Autodesk Inventor part; units mm, degrees
ref_plane "YZ Plane" through (0, 0, 0) normal (1, 0, 0) x (0, 1, 0)
ref_plane "XZ Plane" through (0, 0, 0) normal (0, 1, 0) x (-1, 0, 0)
ref_plane "XY Plane" through (0, 0, 0) normal (0, 0, 1) x (1, 0, 0)
sketch "Sketch1" plane through (0, 0, 0) normal (0, 0, 1) x (1, 0, 0)
  circle A0 centre (15, -15) radius 1.2295
  circle A1 centre (-15, 15) radius 1.2295
  circle A2 centre (15, 15) radius 1.2295
  circle A3 centre (-15, -15) radius 1.2295
  line L0 (-15.5, -17.5) -> (-17.5, -15.5)
  line L1 (-15.5, -17.5) -> (15.5, -17.5)
  line L2 (17.5, -15.5) -> (15.5, -17.5)
  line L3 (17.5, -15.5) -> (17.5, 15.5)
  line L4 (15.5, 17.5) -> (17.5, 15.5)
  line L5 (15.5, 17.5) -> (-15.5, 17.5)
  line L6 (-17.5, 15.5) -> (-15.5, 17.5)
  line L7 (-17.5, 15.5) -> (-17.5, -15.5)
  point P0 (0, 0)
  point P1 (0, 0)
  point P2 (0, 0)
extrude "Extrusion1" add sketch "Sketch1" along normal mid plane 7.5
sketch "Sketch4" plane through (0, 0, -3.75) normal (0, 0, -1) x (-1, 0, 0)
  line L0 (-13.25, 13.25) -> (13.25, 13.25)
  line L1 (13.25, 13.25) -> (13.25, -13.25)
  line L2 (13.25, -13.25) -> (-13.25, -13.25)
  line L3 (-13.25, -13.25) -> (-13.25, 13.25)
  line L4 (-17.5, 15.5) -> (-17.5, -15.5)
  line L5 (15.5, 17.5) -> (-15.5, 17.5)
  point P0 (0, 0)
  point P1 (-13.25, 0)
  point P2 (0, 13.25)
  dimension "d15" = 4.25
  dimension "d16" = 4.25
extrude "Extrusion4" add sketch "Sketch4" along normal blind 12.5
sketch "Sketch5" plane through (0, 0, 3.75) normal (0, 0, 1) x (1, 0, 0)
  line L0 (13.25, -13.25) -> (-13.25, -13.25)
  line L1 (-13.25, -13.25) -> (-13.25, 13.25)
  line L2 (-13.25, 13.25) -> (13.25, 13.25)
  line L3 (13.25, 13.25) -> (13.25, -13.25)
  line L4 (-11.25, -11.25) -> (11.25, -11.25)
  line L5 (11.25, -11.25) -> (11.25, 11.25)
  line L6 (11.25, 11.25) -> (-11.25, 11.25)
  line L7 (-11.25, 11.25) -> (-11.25, -11.25)
  point P0 (0, 0)
  dimension "d19" = 2
extrude "Extrusion5" cut sketch "Sketch5" against normal blind 12.5 contours L7 L6 L5 L4
fillet "Fillet2" radius 2 4 edges at (11.25, 0, 3.75) (-11.25, 0, 3.75) (0, 11.25, 3.75) (0, -11.25, 3.75)
chamfer "Chamfer2" distance 2 angle 45 8 edges at (13.25, -13.25, -10) (13.25, 13.25, -10) (-13.25, -13.25, -10) (-13.25, 13.25, -10) (0, -13.25, -16.25) (13.25, 0, -16.25) (0, 13.25, -16.25) (-13.25, 0, -16.25)
fillet "Fillet3" radius 2 8 edges at (13.25, 0, -3.75) (12.25, 12.25, -3.75) (0, 13.25, -3.75) (-12.25, 12.25, -3.75) (-13.25, 0, -3.75) (-12.25, -12.25, -3.75) (0, -13.25, -3.75) (12.25, -12.25, -3.75)
properties part number "Back cover for servo motor 250 W" material "PBT Plastic"
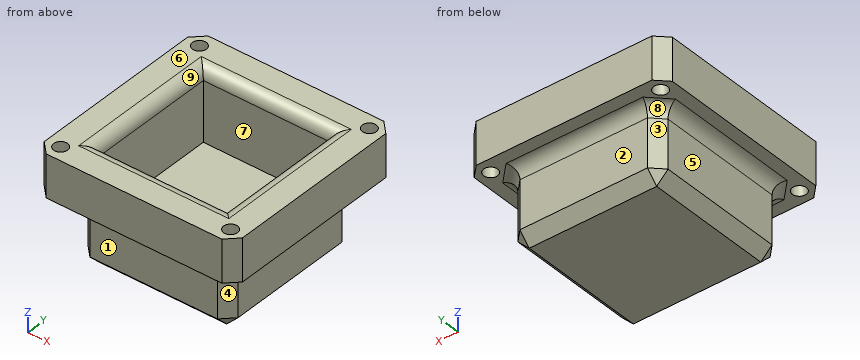
Source: CAD feature listing. Evaluate the final solid. Frame: model axes, mm. Face numbers are marked on the shaded views. A direction names the side the tool comes from. Give positions to 0.01 mm unless a question says otherwise; leave off trailing zeros. Write each loop counter-clockwise with the first axis right and the second up, starting at its lowest first coordinate (ties: lowest second). Pieces come first, ordered by that corner, then holes. Notation, with made-up numbers: M -15.5,62 L 19.5,62 A20 cw 19.5,81 Z; hole C 80.25,-1 d5. An arc over 180 degrees is marked long. Return JSON: item names as keys, results as strings. Group by question number.
1) Pin query (flat end, axial travel): P1, Ø2, axis at x = -15, y = 15, coming from the -Z side; P2, Ø11, axis at x = 0, y = -3.5, coming from the +Z side; P3, Ø4, axis at y = 0.5, z = -11, coming from the -X side; P4, Ø4, axis at y = -2.5, z = -11.5, coming from the +X side. Return the tip coordinate at first contact, or that it passes through.
2) Cut plane C-C, the plane z = 1.25. Output: boundary loops of the cut face in (x, y).
3) Material intervals for line 1 along Y through (x, z) = (-15, 1.25); line 2 along Y through (x, z) = (4, 1.75), sorted ascending. Write a range as [from, to].
4) Set-up query: the marked faces 1, 2, 3, 4 and 5. Return all of +Z, -Z, +X, -X, +Y, -Y with unobstructed straight access to the full face (end or side cutting, diameter ignored); none if empty.
5) Cut plane A-A, the plane z = -6.5. Output: boundary loops of the cut face in (x, y).
6) Pull-direction query (Y, two-part tool) for the marked faces 6, 7, 8 and 9; classes: pulls with the +Y half, pulls with the -Y half, needs draft (parallel to the pull), parting line crosses it, or undercut.
7) Cut plane B-B, the plane x = 2. Output: boundary loops of the cut face in (y, z), plus the area to 4 significant figures.
Recorded:
{
 "1": {"P1": "passes through", "P2": "stops at z = -8.75", "P3": "stops at x = -13.25", "P4": "stops at x = 13.25"},
 "2": {"outline": "M -17.5,-15.5 L -15.5,-17.5 L 15.5,-17.5 L 17.5,-15.5 L 17.5,15.5 L 15.5,17.5 L -15.5,17.5 L -17.5,15.5 Z; hole C -15,-15 d2.46; hole C -15,15 d2.46; hole M -11.25,-11.25 L 11.25,-11.25 L 11.25,11.25 L -11.25,11.25 Z; hole C 15,-15 d2.46; hole C 15,15 d2.46"},
 "3": {"line 1": "y = [-17.5, -16.23], [-13.77, 13.77], [16.23, 17.5]", "line 2": "y = [-17.5, -11.25], [11.25, 17.5]"},
 "4": {"face 1": "-Z, +X, -X, -Y", "face 2": "-Z, +X, -X, +Y", "face 3": "-Z, -X, +Y", "face 4": "-Z, +X, -Y", "face 5": "-Z, -X, +Y, -Y"},
 "5": {"outline": "M -13.25,-11.25 L -11.25,-13.25 L 11.25,-13.25 L 13.25,-11.25 L 13.25,11.25 L 11.25,13.25 L -11.25,13.25 L -13.25,11.25 Z; hole M -11.25,-11.25 L 11.25,-11.25 L 11.25,11.25 L -11.25,11.25 Z"},
 "6": {"face 6": "needs draft", "face 7": "undercut", "face 8": "pulls with the +Y half", "face 9": "undercut"},
 "7": {"outline": "M -17.5,-3.75 L -15.25,-3.75 A2 cw -13.25,-5.75 L -13.25,-14.25 L -11.25,-16.25 L 11.25,-16.25 L 13.25,-14.25 L 13.25,-5.75 A2 cw 15.25,-3.75 L 17.5,-3.75 L 17.5,3.75 L 13.25,3.75 A2 ccw 11.25,1.75 L 11.25,-8.75 L -11.25,-8.75 L -11.25,1.75 A2 ccw -13.25,3.75 L -17.5,3.75 Z", "area": "308.5 mm²"}
}
